```python
from build123d import *

# Parameters (mm, degrees)
F0_W     = 10
F0_H     = 40.3
F0_W_2   = 4.6593984449
F0_H_2   = 28.3
F1_DEPTH = 17
F2_DEPTH = 9


# Not quite as in the source:
# - a feature names something its author has since deleted; it is built from what else it names


with BuildPart() as f1:
    # F0 (on Front) → F1 (new body)
    with BuildSketch(Plane.XZ):
        with Locations((-25.2545091997, -60.7344553381)):
            Rectangle(F0_W, F0_H)
        with Locations((-25.3930282849, -60.7344553381)):
            Rectangle(F0_W_2, F0_H_2, mode=Mode.SUBTRACT)
        with Locations((-25.3930282849, -60.7344553381)):
            Rectangle(F0_W_2, F0_H_2)
    extrude(amount=F1_DEPTH)

    # F0 (on Front) → F2 (cut)
    with BuildSketch(Plane.XZ):
        with Locations((-25.3930282849, -60.7344553381)):
            Rectangle(F0_W_2, F0_H_2)
    extrude(amount=F2_DEPTH, mode=Mode.SUBTRACT)


solid = f1.part
```
Geometry: final body of the model. Coordinates: model frame, mm. A direction names the side the tool comes from. Round coordinates to 2 decimals unless told otherwise and drop trailing zeros. Loops run counter-clockwise (first coordinate to the right, second up) from the corner with the lowest first, then second, coordinate; pieces in that order, holes last. Notation, with made-up numbers: (-21.5, 82.5) -> (12.5, 82.5) arc R23 cw to (12.5, 120.5) -> close; hole circle Ø1 at (4, 47.25). An arc over 180 degrees is marked (long way). Use one line per item in the form item = value. Start each with the question number.
1) Draft query along Z for faces 3 (the flat face through (-25, -4, -74.884)), 4 (the flat face through (-25, -8, -80.884)), 5 (the flat face through (-22, 0, -60)). Return one class per face: released by +Z, released by -Z, zero draft, split by the parting line, or undercut.
2) Access query for faces 1 (the flat face through (-25, -17, -60)), 2 (the flat face through (-25, -9, -61)). Directions: +Z, -Z, +X, -X, +Y, -Y. A direction counts if a zero-diameter tool reaches every point of the face in a straight line with its end or side. Return the directions, or none.
3) Section C-C on x = -25. Output: boundary loops of the cut face in (y, z), then the cut area to 3 significant figures.
4) First-contact query: P1, Ø1.4, axis at x = -26, z = -56.5, coming from the +Y side. Flat tip, straight axial feed; report the tip coordinate or a pass-through.
5) Section A-A on y = -6. Output: boundary loops of the cut face in (x, z), then the cut area to 3 significant figures.
6) Line query: L1, parallel to X at y = -4.25, z = -53; L2, parallel to Z at x = -25.75, y = -8.75; L3, parallel to Y at x = -26.75, z = -64. Output: solid intervals per line, ascending.
7) Section B-B on z = -73.5. Output: boundary loops of the cut face in (x, y), then the cut area to 3 significant figures.
Response:
q1.face_3 = undercut
q1.face_4 = released by -Z
q1.face_5 = zero draft
q2.face_1 = +Z, -Z, +X, -X, -Y
q2.face_2 = +Y
q3.outline = (-17, -80.88) -> (0, -80.88) -> (0, -74.88) -> (-9, -74.88) -> (-9, -46.58) -> (0, -46.58) -> (0, -40.58) -> (-17, -40.58) -> close
q3.area = 430 mm^2
q4.P1 = -9
q5.outline = (-30.25, -80.88) -> (-20.25, -80.88) -> (-20.25, -40.58) -> (-30.25, -40.58) -> close; hole (-27.72, -74.88) -> (-23.06, -74.88) -> (-23.06, -46.58) -> (-27.72, -46.58) -> close
q5.area = 271 mm^2
q6.L1 = -30.25 to -27.72, -23.06 to -20.25
q6.L2 = -80.88 to -74.88, -46.58 to -40.58
q6.L3 = -17 to -9
q7.outline = (-30.25, -17) -> (-20.25, -17) -> (-20.25, 0) -> (-23.06, 0) -> (-23.06, -9) -> (-27.72, -9) -> (-27.72, 0) -> (-30.25, 0) -> close
q7.area = 128 mm^2
